Study the drawing (mm; zero at the part's minimum x, y, z) and answer. A direction names the side the tool comes from. Round coordinates to 2 decimals unless told otherwise and drop trailing zeros. Write each loop counter-clockwise with the first axis right and the second up, starting at its lowest first coordinate (ties: lowest second). Pieces come first, ordered by that corner, then holes.
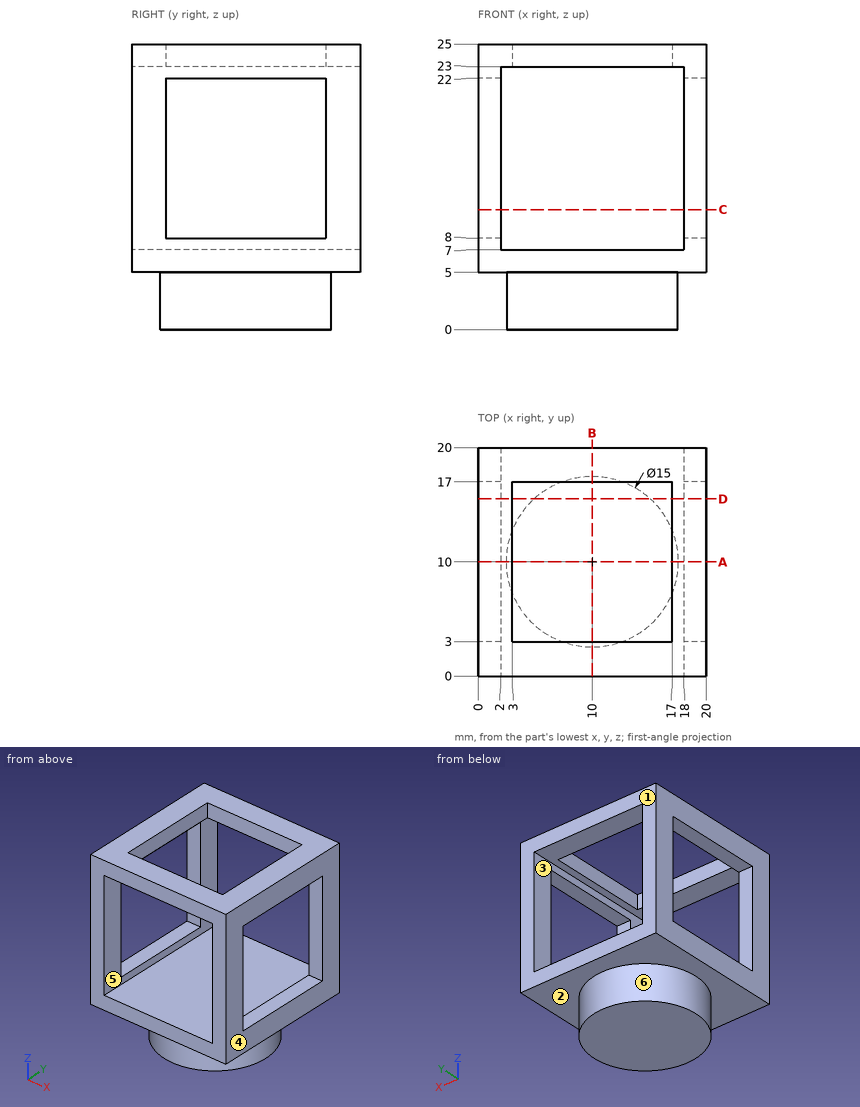
1. Straight lines are drawn through the part: line 1 along Z through (x, y) = (1.5, 11.5); line 2 along Z through (x, y) = (14.75, 2.75); line 3 along X through (y, z) = (17.5, 8.75). For each, find the intervals that lie inside material, in ascending order.
Geometry says:
line 1: z = 5 to 8, 22 to 25
line 2: z = 5 to 7, 23 to 25
line 3: x = 0 to 2, 18 to 20
2. Section D-D on y = 15.5 is taken. Determine the outline of the cut face in (x, z), plus the area to 3 significant figures.
Geometry says:
outline: (0, 5) - (4.9, 5) - (4.9, 0) - (15.1, 0) - (15.1, 5) - (20, 5) - (20, 8) - (18, 8) - (18, 7) - (2, 7) - (2, 8) - (0, 8) - close; (0, 22) - (2, 22) - (2, 23) - (3, 23) - (3, 25) - (0, 25) - close; (17, 23) - (18, 23) - (18, 22) - (20, 22) - (20, 25) - (17, 25) - close
area: 111 mm2
3. A tool of negligible diameter and unlimited length cuts with its end or side. For the marked faces 1, 2 and 3, from which of +Z, -Z, +X, -X, +Y, -Y can it reach the whole face along a straight path? Write none if from no direction.
Geometry says:
face 1: +Z, -Z, +X, -X, +Y
face 2: -Z
face 3: +Y, -Y
4. Section C-C on z = 10.5 is taken. Determine the outline of the cut face in (x, y), plus the area to 3 significant figures.
Geometry says:
outline: (0, 0) - (2, 0) - (2, 3) - (0, 3) - close; (0, 17) - (2, 17) - (2, 20) - (0, 20) - close; (18, 0) - (20, 0) - (20, 3) - (18, 3) - close; (18, 17) - (20, 17) - (20, 20) - (18, 20) - close
area: 24.0 mm2
5. Given pin 1 (5 mm diameter, centred on x = 9.5, y = 9, fed in from +Z), flat-ended and moving along its own axis, determine where the tip first touches the part or whether it passes through.
Geometry says:
pin 1: stops at z = 7
6. For a pull along X with two mould halves and no side action, classify the marked faces 4, 5 and 6 as released by +X, released by -X, zero draft, split by the parting line, or undercut.
Geometry says:
face 4: released by +X
face 5: undercut
face 6: split by the parting line
7. Section A-A on y = 10 is taken. Determine the outline of the cut face in (x, z).
Geometry says:
outline: (0, 5) - (2.5, 5) - (2.5, 0) - (17.5, 0) - (17.5, 5) - (20, 5) - (20, 8) - (18, 8) - (18, 7) - (2, 7) - (2, 8) - (0, 8) - close; (0, 22) - (2, 22) - (2, 23) - (3, 23) - (3, 25) - (0, 25) - close; (17, 23) - (18, 23) - (18, 22) - (20, 22) - (20, 25) - (17, 25) - close
8. Section B-B on x = 10 is taken. Determine the outline of the cut face in (y, z), plus the area to 3 significant figures.
Geometry says:
outline: (0, 5) - (2.5, 5) - (2.5, 0) - (17.5, 0) - (17.5, 5) - (20, 5) - (20, 7) - (0, 7) - close; (0, 23) - (3, 23) - (3, 25) - (0, 25) - close; (17, 23) - (20, 23) - (20, 25) - (17, 25) - close
area: 127 mm2
